Can you work these out from the model? Positions are in its coordinate system, mm. A direction names the side the tool comes from. Coordinates: 2 decimals unless noted, no trailing zeros. Order: outer loops, then holes, each group sorted by start corner. A loop starts at its lowest first (then second) coordinate and runs counter-clockwise, first axis right, second up. Notation, with made-up numbers: (-17.75, 59.5) - (9.25, 59.5) arc R5 ccw to (9.25, 66.5) - close; hole circle Ø4 at (-15.75, -13.5). An arc over 180 degrees is marked (long way). Use a Markdown table: item, result. Add a question column.
(1) On a 3-axis mill with a long thin cutter (end or side, diameter ignored), from which of +Z, -Z, +X, -X, +Y, -Y can I reach the whole of each face in a straight line? I mean faces 1 (the flat face through (-9, 5, -6)), 2 (the flat face through (14, 5, -4.422)), 3 (the flat face through (-8, 1.5, -27)), 4 (the cylindrical face through (-11.089, 5.814, -2.45)), 5 (the flat face through (0, 0, -10)). Say none if no direction works.
(2) I want a section at D-D (z = -21.5). List the corners of the cut face in (x, y) for me, and give its area (3 significant figures).
(3) If I drill on L1, parallel to Z at x = 0, y = 0.5; L2, parallel to Z at x = -9.5, y = 2.5; L3, parallel to X at y = 6.5, z = -20.5, over which ranges is the centre line in solid material (lowest first)? Write a range as [from, to].
(4) I want a section at A-A (x = 0). List the corners of the cut face in (y, z) for me.
(5) I want a section at C-C (x = -12.5). List the corners of the cut face in (y, z) for me, and give its area (3 significant figures).
(6) For pin 1 Ø7 at (x, z) = (-3, -25.5) entering from +Y; pin 2 Ø1.3 at (y, z) = (4, -6) entering from +X; pin 3 Ø1.9 at (x, y) = (12.25, 4.75) entering from +Z; pin 4 Ø0.5 at (y, z) = (7, -6.5) entering from -X, each with a flat end and sliding along its axis, tell me the tip position at first contact or that it passes through.
(7) I want a section at B-B (y = 4.75). List the corners of the cut face in (x, z) for me (3 decimals).
(8) We'd pull the mould along X, two halves only. Please class faces 6 (the flat face through (17, 5, -2)), 7 (the cylindrical face through (-0.506, 4.684, -35.414)), 8 (the cylindrical face through (-1.302, 0.74, -10.507)), 9 (the flat face through (0, 9.5, -7)): pulls with the +X half, pulls with the -X half, needs draft (parallel to the pull), parting line crosses it, or undercut.
```python
from build123d import *

# Parameters (mm, degrees)
SKETCH3_R           = 11.25
BOSS_EXTRUDE5_DEPTH = 9.5
SKETCH11_R          = 11.25
SKETCH11_R_2        = 10
BOSS_EXTRUDE6_DEPTH = 1.5
SKETCH12_R          = 1.575
CUT_EXTRUDE3_DEPTH  = 5
SKETCH13_R          = 1.575
CUT_EXTRUDE4_DEPTH  = 5
FILLET1_R           = 3
FILLET1_2_R         = 1


with BuildPart() as part:
    # Sketch3 → Boss-Extrude5 (new body)
    with BuildSketch(Plane(origin=(0, 0, 0), x_dir=(1, 0, 0), z_dir=(0, 1, 0))):
        with BuildLine():
            Line((-15.5, 4.422205102), (-9, 4.422205102))
            Line((-9, 4.422205102), (-9, 8.422205102))
            ThreePointArc((-9, 8.422205102), (0, 35.422205102), (9, 8.422205102))
            Line((9, 8.422205102), (9, 4.422205102))
            Line((9, 4.422205102), (15.5, 4.422205102))
            ThreePointArc((15.5, 4.422205102), (16.560660172, 3.982865274), (17, 2.922205102))
            Line((17, 2.922205102), (17, 0.422205102))
            Line((17, 0.422205102), (-17, 0.422205102))
            Line((-17, 0.422205102), (-17, 2.922205102))
            ThreePointArc((-17, 2.922205102), (-16.560660172, 3.982865274), (-15.5, 4.422205102))
        make_face()
        with Locations((0, 20.422205102)):
            Circle(SKETCH3_R, mode=Mode.SUBTRACT)
    extrude(amount=BOSS_EXTRUDE5_DEPTH)

    # Sketch11 → Boss-Extrude6 (add)
    with BuildSketch(Plane.XZ):
        with Locations((0, -20.422205102)):
            Circle(SKETCH11_R)
        with Locations((0, -20.422205102)):
            Circle(SKETCH11_R_2, mode=Mode.SUBTRACT)
    extrude(amount=-BOSS_EXTRUDE6_DEPTH)

    # Sketch12 → Cut-Extrude3 (cut, through all)
    with BuildSketch(Plane(origin=(0, 0, -4.422205102), x_dir=(-1, 0, 0), z_dir=(0, 0, -1))):
        with Locations((12.25, 4.75)):
            Circle(SKETCH12_R)
    extrude(amount=-CUT_EXTRUDE3_DEPTH, mode=Mode.SUBTRACT)

    # Sketch13 → Cut-Extrude4 (cut, through all)
    with BuildSketch(Plane(origin=(0, 0, -4.422205102), x_dir=(-1, 0, 0), z_dir=(0, 0, -1))):
        with Locations((-12.25, 4.75)):
            Circle(SKETCH13_R)
    extrude(amount=-CUT_EXTRUDE4_DEPTH, mode=Mode.SUBTRACT)

    # Fillet1
    fillet1_edges = [part.edges().sort_by_distance(p)[0] for p in [
        (-9, 4.75, -8.422205102),
        (9, 4.75, -8.422205102),
    ]]
    fillet(fillet1_edges, radius=FILLET1_R)

    # Fillet1 2
    fillet1_2_edges = [part.edges().sort_by_distance(p)[0] for p in [
        (-9, 4.75, -4.422205102),
        (9, 4.75, -4.422205102),
    ]]
    fillet(fillet1_2_edges, radius=FILLET1_2_R)


solid = part.part
```
Answers follow:
| question | item | result |
|---|---|---|
| 1 | face 1 | -X, +Y, -Y |
| 1 | face 2 | +X, +Y, -Y |
| 1 | face 3 | +Y |
| 1 | face 4 | +Z |
| 1 | face 5 | +Z, -Z, +X, -X, -Y |
| 2 | outline | (-14.96, 0) - (-9.94, 0) - (-9.94, 1.5) - (-11.2, 1.5) - (-11.2, 9.5) - (-14.96, 9.5) - close; (9.94, 0) - (14.96, 0) - (14.96, 9.5) - (11.2, 9.5) - (11.2, 1.5) - (9.94, 1.5) - close |
| 2 | area | 75.3 mm² |
| 3 | L1 | z = [-35.42, -30.42], [-10.42, -0.42] |
| 3 | L2 | z = [-32.03, -26.45], [-14.4, -8.66], [-4.56, -0.42] |
| 3 | L3 | x = [-15, -11.25], [11.25, 15] |
| 4 | outline | (0, -35.42) - (9.5, -35.42) - (9.5, -31.67) - (1.5, -31.67) - (1.5, -30.42) - (0, -30.42) - close; (0, -10.42) - (1.5, -10.42) - (1.5, -9.17) - (9.5, -9.17) - (9.5, -0.42) - (0, -0.42) - close |
| 5 | outline | (0, -28.71) - (9.5, -28.71) - (9.5, -12.13) - (0, -12.13) - close; (0, -4.42) - (3.19, -4.42) - (3.19, -0.42) - (0, -0.42) - close; (6.31, -4.42) - (9.5, -4.42) - (9.5, -0.42) - (6.31, -0.42) - close |
| 5 | area | 183 mm² |
| 6 | pin 1 | passes through |
| 6 | pin 2 | stops at x = 9 |
| 6 | pin 3 | stops at z = -10.56 |
| 6 | pin 4 | stops at x = -9 |
| 7 | outline | (-17, -2.922) arc R1.5 ccw to (-15.5, -4.422) - (-13.825, -4.422) - (-13.825, -0.422) - (-17, -0.422) - close; (-10.675, -4.422) - (-10, -4.422) arc R1 cw to (-9, -5.422) - (-9, -7.006) arc R3 cw to (-10, -9.242) arc R15 ccw (long way) to (10, -9.242) arc R3 cw to (9, -7.006) - (9, -5.422) arc R1 cw to (10, -4.422) - (10.675, -4.422) - (10.675, -0.422) - (-10.675, -0.422) - close; (13.825, -4.422) - (15.5, -4.422) arc R1.5 ccw to (17, -2.922) - (17, -0.422) - (13.825, -0.422) - close; hole circle Ø22.5 at (0, -20.422) |
| 8 | face 6 | pulls with the +X half |
| 8 | face 7 | parting line crosses it |
| 8 | face 8 | undercut |
| 8 | face 9 | needs draft |
